Input: dimensioned drawing with shaded views. Units: mm. Origin: part minimum x, y, z. Round coordinates to 2 decimals unless told otherwise and drop trailing zeros. Order: outer loops, then holes, each group sorted by start corner. A loop starts at its lowest first (then second) coordinate and runs counter-clockwise, first axis right, second up. Notation, with made-up numbers: (-32, 2.5) - (16, 2.5) arc R18 ccw to (16, 17.5) - close; hole circle Ø3 at (-13.75, 71.5). An arc over 180 degrees is marked (long way). Put each result on its own line as item: value. Start each with the question number.
(1) Section C-C (y = 41). Output: boundary loops of the cut face in (x, z) (1 decimal), and give its area (3 significant figures).
(2) Material intervals for L1, parallel to Y at x = 19, z = 3.05; L2, parallel to X at y = 64, z = 2.4; L3, parallel to Y at x = 20.5, z = 1.55 (1 decimal), sorted ascending. Write a range as [from, to].
(3) Section A-A (x = 19.05). Output: boundary loops of the cut face in (y, z) (1 decimal).
(4) Section B-B (z = 0.85). Output: boundary loops of the cut face in (x, y).
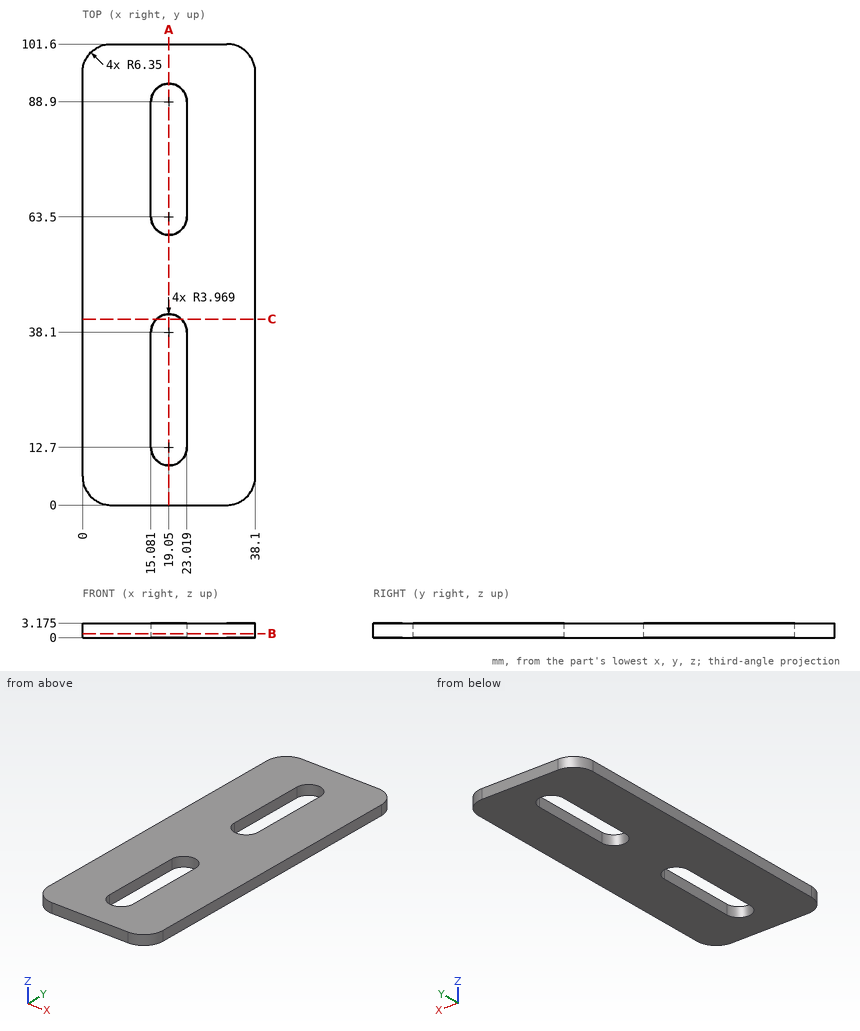
Checks:
1. outline: (0, 0) - (16.3, 0) - (16.3, 3.2) - (0, 3.2) - close; (21.8, 0) - (38.1, 0) - (38.1, 3.2) - (21.8, 3.2) - close
1. area: 104 mm²
2. L1: y = [0, 8.73], [42.07, 59.53], [92.87, 101.6]
2. L2: x = [0, 15.08], [23.02, 38.1]
2. L3: y = [0, 9], [41.8, 59.8], [92.6, 101.6]
3. outline: (0, 0) - (8.7, 0) - (8.7, 3.2) - (0, 3.2) - close; (42.1, 0) - (59.5, 0) - (59.5, 3.2) - (42.1, 3.2) - close; (92.9, 0) - (101.6, 0) - (101.6, 3.2) - (92.9, 3.2) - close
4. outline: (0, 6.35) arc R6.35 ccw to (6.35, 0) - (31.75, 0) arc R6.35 ccw to (38.1, 6.35) - (38.1, 95.25) arc R6.35 ccw to (31.75, 101.6) - (6.35, 101.6) arc R6.35 ccw to (0, 95.25) - close; hole (15.08, 12.7) arc R3.97 ccw to (23.02, 12.7) - (23.02, 38.1) arc R3.97 ccw to (15.08, 38.1) - close; hole (15.08, 63.5) arc R3.97 ccw to (23.02, 63.5) - (23.02, 88.9) arc R3.97 ccw to (15.08, 88.9) - close
